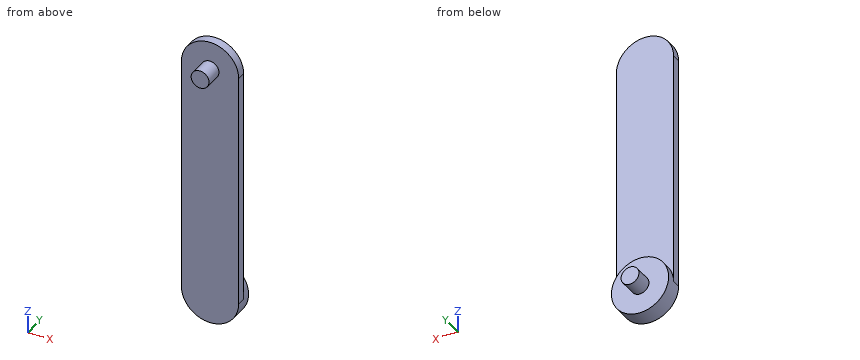
from build123d import *

# Parameters (mm, degrees)
BOSS_EXTRUDE1_DEPTH = 2.5
BOSS_EXTRUDE5_DEPTH = 1.25
SKETCH4_R           = 1.25
BOSS_EXTRUDE6_DEPTH = 2.5
SKETCH5_R           = 1.25
BOSS_EXTRUDE7_DEPTH = 2.5


with BuildPart() as part:
    # Sketch1 → Boss-Extrude1 (new body)
    with BuildSketch(Plane(origin=(0, 0, 0), x_dir=(1, 0, 0), z_dir=(0, 1, 0))):
        with BuildLine():
            ThreePointArc((4, 33), (0, 37), (-4, 33))
            ThreePointArc((-4, 33), (0, 29), (4, 33))
        make_face()
    extrude(amount=BOSS_EXTRUDE1_DEPTH)

    # Sketch1<5> → Boss-Extrude5 (add)
    with BuildSketch(Plane(origin=(0, 0, 0), x_dir=(1, 0, 0), z_dir=(0, 1, 0))):
        with BuildLine():
            Line((-4, 33), (-4, 0))
            ThreePointArc((-4, 0), (0, -4), (4, 0))
            Line((4, 0), (4, 33))
            ThreePointArc((4, 33), (0, 29), (-4, 33))
        make_face()
    extrude(amount=BOSS_EXTRUDE5_DEPTH)

    # Sketch4 → Boss-Extrude6 (add)
    with BuildSketch(Plane(origin=(0, 2.5, 0), x_dir=(1, 0, 0), z_dir=(0, 1, 0))):
        with Locations((0, 33)):
            Circle(SKETCH4_R)
    extrude(amount=BOSS_EXTRUDE6_DEPTH)

    # Sketch5 → Boss-Extrude7 (add)
    with BuildSketch(Plane.XZ):
        Circle(SKETCH5_R)
    extrude(amount=BOSS_EXTRUDE7_DEPTH)


solid = part.part
Geometry check sheet. Reference: the model listing, model coordinates, mm. Round coordinates to 2 decimals unless told otherwise and drop trailing zeros. Order: outer loops, then holes, each group sorted by start corner. A loop starts at its lowest first (then second) coordinate and runs counter-clockwise, first axis right, second up. Notation, with made-up numbers: (22.25, 68.5) - (40.25, 68.5) arc R29 ccw to (40.25, 90.5) - close; hole circle Ø4 at (31.25, -12.75). An arc over 180 degrees is marked (long way). One line per question, with ' | ' between items. Start each with the question number.
(1) Depth check by flat-ended pin: pin 1 Ø3 at (x, y) = (2, 2.5) entering from -Z; pin 2 Ø4 at (x, y) = (2, 2) entering from +Z; pin 3 Ø4 at (x, z) = (-1, -34.5) entering from +Y; pin 4 Ø1 at (x, y) = (2, 0.5) entering from -Z. Enter the tip coordinate at first touch or a pass-through.
(2) Sectioned sample at B-B on z = -7.5. Record the cut outline in (x, y), and give its area (3 significant figures).
(3) Sectioned sample at A-A on x = -0.75. Record the cut outline in (y, z), and give its area (3 significant figures).
(4) Sectioned sample at C-C on y = 3.75. Record the cut outline in (x, z), and give its area (3 significant figures).
(5) Sectioned sample at D-D on x = -3. Record the cut outline in (y, z), and give its area (3 significant figures).
(6) Thickness scan on L1, parallel to Y at x = -2.75, z = 1.5; L2, parallel to Y at x = 3, z = -34.5; L3, parallel to Z at x = -3, y = 0.25. Record the ranges inside material, lowest first. Write a range as [from, to].
Conclusion:
1) pin 1: stops at z = -36.97 | pin 2: stops at z = 4 | pin 3: stops at y = 5 | pin 4: stops at z = -36.71
2) outline: (-4, 0) - (4, 0) - (4, 1.25) - (-4, 1.25) - close | area: 10.0 mm2
3) outline: (-2.5, -1) - (0, -1) - (0, -36.93) - (2.5, -36.93) - (2.5, -34) - (5, -34) - (5, -32) - (2.5, -32) - (2.5, -29.07) - (1.25, -29.07) - (1.25, 3.93) - (0, 3.93) - (0, 1) - (-2.5, 1) - close | area: 70.9 mm2
4) outline: circle Ø2.5 at (0, -33) | area: 4.91 mm2
5) outline: (0, -35.65) - (2.5, -35.65) - (2.5, -30.35) - (1.25, -30.35) - (1.25, 2.65) - (0, 2.65) - close | area: 54.5 mm2
6) L1: y = [0, 1.25] | L2: y = [0, 2.5] | L3: z = [-35.65, 2.65]
